Here's how the part is built. I have some questions about the finished solid (model axes, mm). Face numbers are marked on the shaded views. A direction names the side the tool comes from. Coordinates: 2 decimals unless noted, no trailing zeros. Order: outer loops, then holes, each group sorted by start corner. A loop starts at its lowest first (then second) coordinate and runs counter-clockwise, first axis right, second up. Notation, with made-up numbers: M 34.5,-13.5 L 46.5,-13.5 A20 ccw 46.5,8.5 Z; hole C 40.25,-22 d3. An arc over 180 degrees is marked long. One line per question, with ' | ' between items. Start each with the question number.
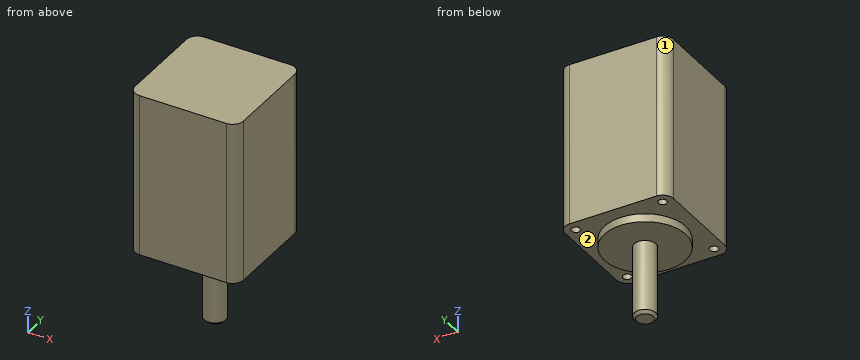
```python
from build123d import *

# Parameters (mm, degrees)
SKETCH1_W                 = 20
SKETCH1_H                 = 20
BOSS_EXTRUDE1_DEPTH       = 30
SKETCH2_R                 = 7.5
BOSS_EXTRUDE2_DEPTH       = 1.5
SKETCH3_R                 = 2
BOSS_EXTRUDE3_DEPTH       = 13.5
M2X0_4_TAPPED_HOLE1_D     = 1.6
M2X0_4_TAPPED_HOLE1_DEPTH = 3.5
M2X0_4_TAPPED_HOLE1_TIP   = 0.480688495
FILLET1_R                 = 2
CHAMFER1_SIZE             = 0.5


with BuildPart() as part:
    # Sketch1 → Boss-Extrude1 (new body)
    with BuildSketch(Plane.XY):
        Rectangle(SKETCH1_W, SKETCH1_H)
    extrude(amount=BOSS_EXTRUDE1_DEPTH)

    # Sketch2 → Boss-Extrude2 (add)
    with BuildSketch(Plane(origin=(0, 0, 0), x_dir=(-1, 0, 0), z_dir=(0, 0, -1))):
        Circle(SKETCH2_R)
    extrude(amount=BOSS_EXTRUDE2_DEPTH)

    # Sketch3 → Boss-Extrude3 (add)
    with BuildSketch(Plane(origin=(0, 0, -1.5), x_dir=(-1, 0, 0), z_dir=(0, 0, -1))):
        Circle(SKETCH3_R)
    extrude(amount=BOSS_EXTRUDE3_DEPTH)

    # M2x0.4 Tapped Hole1
    with Locations(Plane(origin=(0, 0, 0), x_dir=(-1, 0, 0), z_dir=(0, 0, -1))):
        with Locations((-8, 8), (8, 8), (8, -8), (-8, -8)):
            Hole(M2X0_4_TAPPED_HOLE1_D / 2, depth=M2X0_4_TAPPED_HOLE1_DEPTH)
            with Locations((0, 0, -(M2X0_4_TAPPED_HOLE1_DEPTH + M2X0_4_TAPPED_HOLE1_TIP / 2))):  # 118° drill point
                Cone(0, M2X0_4_TAPPED_HOLE1_D / 2, M2X0_4_TAPPED_HOLE1_TIP, mode=Mode.SUBTRACT)

    # Fillet1
    fillet1_edges = [part.edges().sort_by_distance(p)[0] for p in [
        (10, -10, 15),
        (-10, -10, 15),
        (-10, 10, 15),
        (10, 10, 15),
    ]]
    fillet(fillet1_edges, radius=FILLET1_R)

    # Chamfer1
    chamfer1_edges = [part.edges().sort_by_distance(p)[0] for p in [
        (2, 0, -15),
    ]]
    chamfer(chamfer1_edges, length=CHAMFER1_SIZE)


solid = part.part
```
1. Imagine slicing it at D-D (z = -10). List the corners of the cut face in (x, y) for me, then the cut area to 3 significant figures.
2. Imagine slicing it at C-C (y = -4.5). List the corners of the cut face in (x, z) for me, then the cut area to 3 significant figures.
3. Imagine slicing it at A-A (y = 0). List the corners of the cut face in (x, z) for me.
4. Which directions (+Z, -Z, +X, -X, +Y, -Y) give clear straight access to the entire face, cutting with the end or side of a thin tool? Please do the marked faces 1 and 2.
5. I need wall thicknesses on line 1 (X direction, y = 8, z = 1.05); line 2 (Z direction, x = 3.25, y = 3.75). Which ranges of each line are inside material? Lowest first, please.
6. Will these pins go through, and if not, where does the flat tip stop? pin 1 (8 mm diameter, centred on y = 3.5, z = -5, fed in from +X); pin 2 (2 mm diameter, centred on x = -6.5, y = -3.5, fed in from -Z); pin 3 (2 mm diameter, centred on x = 8, y = 8, fed in from -Z); pin 4 (8 mm diameter, centred on x = 4, y = -2.5, fed in from -Z).
Entries:
1) outline: C 0,0 d4 | area: 12.6 mm²
2) outline: M -10,0 L -6,0 L -6,-1.5 L 6,-1.5 L 6,0 L 10,0 L 10,30 L -10,30 Z | area: 618 mm²
3) outline: M -10,0 L -7.5,0 L -7.5,-1.5 L -2,-1.5 L -2,-14.5 L -1.5,-15 L 1.5,-15 L 2,-14.5 L 2,-1.5 L 7.5,-1.5 L 7.5,0 L 10,0 L 10,30 L -10,30 Z
4) face 1: +Z, -Z, -X, +Y | face 2: -Z
5) line 1: -10 to -8.8, -7.2 to 7.2, 8.8 to 10 | line 2: -1.5 to 30
6) pin 1: x = 7.34 | pin 2: z = -1.5 | pin 3: z = 0 | pin 4: z = -15
